Check sheet for the drawn part. Datum: minimum x, y, z corner. Units: mm. Give positions to 0.01 mm unless a question says otherwise; leave off trailing zeros. Write each loop counter-clockwise with the first axis right and the second up, starting at its lowest first coordinate (ties: lowest second). Pieces come first, ordered by that corner, then holes. Notation, with made-up numbers: (-5, 80.5) - (26, 80.5) arc R12 ccw to (26, 85.5) - close; hole circle Ø2 at (77, -33). An arc over 180 degrees is marked (long way). Answer as a JSON object with one key per item and string values. Group by question number.
Item 1: Sectioned sample at C-C, the plane x = 0.6. Record the boundary of the cut face in (y, z).
Item 2: Sectioned sample at A-A, the plane y = 3.35. Record the boundary of the cut face in (x, z), and give its area (3 significant figures).
Item 3: Sectioned sample at B-B, the plane z = 0.2. Record the boundary of the cut face in (x, y), and give its area (3 significant figures).
Item 4: Scan lines: line 1 along Y through (x, z) = (0.6, 0.3); line 2 along X through (y, z) = (2.45, 0.3); line 3 along Y through (x, z) = (1, 0.55). Record each from-to range of solid material in increasing order. Write a range as [from, to].
Item 5: Sectioned sample at D-D, the plane y = 2. Record the boundary of the cut face in (x, z).
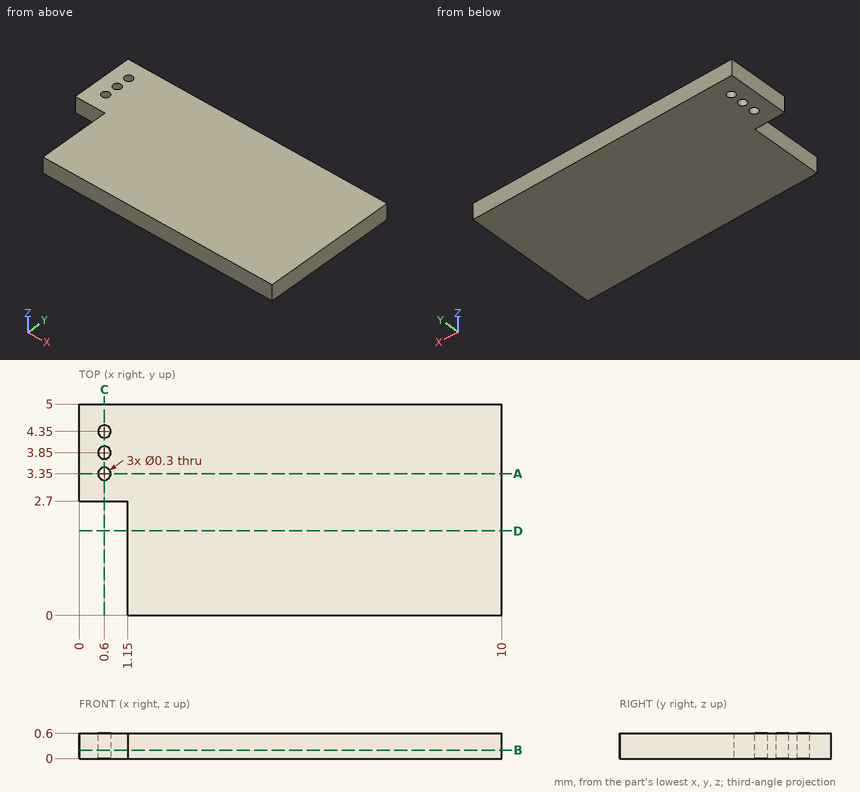
Geometry check:
{
 "1": {"outline": "(2.7, 0) - (3.2, 0) - (3.2, 0.6) - (2.7, 0.6) - close; (3.5, 0) - (3.7, 0) - (3.7, 0.6) - (3.5, 0.6) - close; (4, 0) - (4.2, 0) - (4.2, 0.6) - (4, 0.6) - close; (4.5, 0) - (5, 0) - (5, 0.6) - (4.5, 0.6) - close"},
 "2": {"outline": "(0, 0) - (0.45, 0) - (0.45, 0.6) - (0, 0.6) - close; (0.75, 0) - (10, 0) - (10, 0.6) - (0.75, 0.6) - close", "area": "5.82 mm^2"},
 "3": {"outline": "(0, 2.7) - (1.15, 2.7) - (1.15, 0) - (10, 0) - (10, 5) - (0, 5) - close; hole circle Ø0.3 at (0.6, 3.35); hole circle Ø0.3 at (0.6, 3.85); hole circle Ø0.3 at (0.6, 4.35)", "area": "46.7 mm^2"},
 "4": {"line 1": "[2.7, 3.2], [3.5, 3.7], [4, 4.2], [4.5, 5]", "line 2": "[1.15, 10]", "line 3": "[2.7, 5]"},
 "5": {"outline": "(1.15, 0) - (10, 0) - (10, 0.6) - (1.15, 0.6) - close"}
}
